Part model, mm, in its own coordinate system. A direction names the side the tool comes from. Round coordinates to 2 decimals unless told otherwise and drop trailing zeros. Order: outer loops, then holes, each group sorted by start corner. A loop starts at its lowest first (then second) coordinate and runs counter-clockwise, first axis right, second up. Notation, with made-up numbers: M 42,79 L 88,79 A17 ccw 88,101 Z; hole C -22,53.5 d2. An arc over 180 degrees is marked long. Write each question's results on one line, items separated by ' | '. Start each with the question number.
1. Band-saw the part on B-B, the plane x = -34.5. List the corners of the cut face in (y, z).
2. Which spindle directions (+Z, -Z, +X, -X, +Y, -Y) get a long thin tool onto all of the face, cutting with end or side? Do faces 4 (the face through (-38, -57.15, 35)), 5 (the face through (-38, -31, 0)). Say none if no direction does.
3. Two-plate mould, pull along X, no slides. Class faces 1 (the face through (-7.744, -61.59, 32.106)), 2 (the face through (-37.33, -61.59, 1.81)), 3 (the face through (-12.283, -32, 35)): +X half, -X half, draft (parallel to the pull), parting line (faces both ways), or undercut.
4. Band-saw the part on C-C, the plane y = -19. List the corners of the cut face in (x, z), then the cut area to 3 significant figures.
5. Band-saw the part on A-A, the plane z = 23.5. List the corners of the cut face in (x, y), then the cut area to 3 significant figures.
6. Drop a flat-ended pin along its axis: pin 1 Ø1.5 at (x, y) = (-59.5, -21) entering from +Z. Give the stop position or say it passes through.
7. Band-saw the part on D-D, the plane z = 4.5. List the corners of the cut face in (x, y).
8. Probe L1, parallel to X at y = -25.5, z = 48.5; L2, parallel to Y at x = -33, z = 56.5. List the from-to ranges inside material, lowest first. Write a range as [from, to].
```python
from build123d import *

# Parameters (mm, degrees)
F0_W     = 63.5
F0_H     = 63.5
F1_DEPTH = 63.5
F2_R     = 6.35
F3_W     = 50.8
F3_H     = 50.8
F4_DEPTH = 57.15


with BuildPart() as f1:
    # F0 (on Front) → F1 (new body)
    with BuildSketch(Plane.XZ):
        with Locations((-37.683266, 31.75)):
            Rectangle(F0_W, F0_H)
    extrude(amount=F1_DEPTH)

    # F2
    f2_edges = [f1.edges().sort_by_distance(p)[0] for p in [
        (-69.433266, -31.75, 0),
        (-5.933266, -31.75, 0),
        (-37.683266, 0, 0),
        (-37.683266, -63.5, 0),
        (-37.683266, -63.5, 63.5),
        (-69.433266, -63.5, 31.75),
        (-5.933266, -63.5, 31.75),
        (-5.933266, -31.75, 63.5),
        (-5.933266, 0, 31.75),
        (-37.683266, 0, 63.5),
        (-69.433266, 0, 31.75),
        (-69.433266, -31.75, 63.5),
    ]]
    fillet(f2_edges, radius=F2_R)

    # F3 (on face) → F4 (cut)
    with BuildSketch(Plane.XY.offset(63.5)):
        with Locations((-37.683266, -31.75)):
            Rectangle(F3_W, F3_H)
    extrude(amount=-F4_DEPTH, mode=Mode.SUBTRACT)


solid = f1.part
```
Solution:
1) outline: M -63.5,6.35 A6.35 ccw -57.15,0 L -6.35,0 A6.35 ccw 0,6.35 L 0,57.15 A6.35 ccw -6.35,63.5 L -6.35,6.35 L -57.15,6.35 L -57.15,63.5 A6.35 ccw -63.5,57.15 Z
2) face 4: +Z | face 5: -Z, +X, -X, +Y, -Y
3) face 1: +X half | face 2: draft | face 3: undercut
4) outline: M -69.43,6.35 A6.35 ccw -63.08,0 L -12.28,0 A6.35 ccw -5.93,6.35 L -5.93,57.15 A6.35 ccw -12.28,63.5 L -12.28,6.35 L -63.08,6.35 L -63.08,63.5 A6.35 ccw -69.43,57.15 Z | area: 1,090 mm^2
5) outline: M -69.43,-57.15 A6.35 ccw -63.08,-63.5 L -12.28,-63.5 A6.35 ccw -5.93,-57.15 L -5.93,-6.35 A6.35 ccw -12.28,0 L -63.08,0 A6.35 ccw -69.43,-6.35 Z; hole M -63.08,-57.15 L -12.28,-57.15 L -12.28,-6.35 L -63.08,-6.35 Z | area: 1,420 mm^2
6) pin 1: z = 6.35
7) outline: M -69.16,-57.15 A6.07 ccw -63.08,-63.22 L -12.28,-63.22 A6.07 ccw -6.21,-57.15 L -6.21,-6.35 A6.07 ccw -12.28,-0.28 L -63.08,-0.28 A6.07 ccw -69.16,-6.35 Z
8) L1: [-69.43, -63.08], [-12.28, -5.93] | L2: [-63.5, -57.15], [-6.35, 0]
